Build history of the part. All positions in model axes, mm. A direction names the side the tool comes from. Give positions to 0.01 mm unless a question says otherwise; leave off trailing zeros. Write each loop counter-clockwise with the first axis right and the second up, starting at its lowest first coordinate (ties: lowest second). Pieces come first, ordered by that corner, then holes.
Autodesk Inventor part; units mm, degrees
ref_plane "YZ Plane" through (0, 0, 0) normal (1, 0, 0) x (0, 1, 0)
ref_plane "XZ Plane" through (0, 0, 0) normal (0, 1, 0) x (-1, 0, 0)
ref_plane "XY Plane" through (0, 0, 0) normal (0, 0, 1) x (1, 0, 0)
sketch "Sketch1" plane through (0, 0, 0) normal (0, 1, 0) x (-1, 0, 0)
  line L0 (0, 0) -> (100, 0)
  line L1 (100, 0) -> (100, -180)
  line L2 (100, -180) -> (0, -180)
  line L3 (0, -180) -> (0, 0)
  dimension "d0" = 100
  dimension "d1" = 180
sketch "Sketch2" plane through (0, 0, 0) normal (0, 1, 0) x (-1, 0, 0)
  circle A0 centre (49.0743, -61.8964) radius 10
  circle A1 centre (49.0743, -103.4918) radius 10
  circle A2 centre (49.0743, -145.129) radius 10
  line L0 (82.079, -27.0534) -> (82.079, -47.0534) construction
  line L1 (86.0942, -27.0534) -> (86.0942, -47.0534)
  line L2 (78.0638, -47.0534) -> (78.0638, -27.0534)
  arc A3 (86.0942, -27.0534) -> (78.0638, -27.0534) centre (82.079, -27.0534) ccw
  arc A4 (78.0638, -47.0534) -> (86.0942, -47.0534) centre (82.079, -47.0534) ccw
  line L3 (16.5655, -27.0534) -> (16.5655, -47.0534) construction
  line L4 (20.5808, -27.0534) -> (20.5808, -47.0534)
  line L5 (12.5503, -47.0534) -> (12.5503, -27.0534)
  arc A5 (20.5808, -27.0534) -> (12.5503, -27.0534) centre (16.5655, -27.0534) ccw
  arc A6 (12.5503, -47.0534) -> (20.5808, -47.0534) centre (16.5655, -47.0534) ccw
  line L6 (82.079, -138.3165) -> (82.079, -158.3165) construction
  line L7 (86.0942, -138.3165) -> (86.0942, -158.3165)
  line L8 (78.0638, -158.3165) -> (78.0638, -138.3165)
  arc A7 (86.0942, -138.3165) -> (78.0638, -138.3165) centre (82.079, -138.3165) ccw
  arc A8 (78.0638, -158.3165) -> (86.0942, -158.3165) centre (82.079, -158.3165) ccw
  line L9 (16.5655, -138.3165) -> (16.5655, -158.3165) construction
  line L10 (20.5808, -138.3165) -> (20.5808, -158.3165)
  line L11 (12.5503, -158.3165) -> (12.5503, -138.3165)
  arc A9 (20.5808, -138.3165) -> (12.5503, -138.3165) centre (16.5655, -138.3165) ccw
  arc A10 (12.5503, -158.3165) -> (20.5808, -158.3165) centre (16.5655, -158.3165) ccw
  point P0 (0, 0)
  point P1 (82.079, -37.0534)
  point P2 (16.5655, -37.0534)
  point P3 (82.079, -148.3165)
  point P4 (16.5655, -148.3165)
  dimension "d3" = 20
  dimension "d13" = 20
  dimension "d14" = 20
  dimension "d15" = 20
  dimension "d16" = 20
extrude "Extrusion1" add sketch "Sketch1" along normal blind 10
extrude "Extrusion2" cut sketch "Sketch2" along normal blind 10
sketch "Sketch6" plane through (0, 10, 0) normal (0, 1, 0) x (1, 0, 0)
  line L0 (-48.9569, 12.2049) -> (-48.9569, 32.2049) construction
  line L1 (-43.9569, 12.2049) -> (-43.9569, 32.2049)
  line L2 (-53.9569, 32.2049) -> (-53.9569, 12.2049)
  arc A0 (-53.9569, 12.2049) -> (-43.9569, 12.2049) centre (-48.9569, 12.2049) ccw
  arc A1 (-43.9569, 32.2049) -> (-53.9569, 32.2049) centre (-48.9569, 32.2049) ccw
  point P0 (0, 0)
  point P1 (-48.9569, 22.2049)
  dimension "d9" = 20
extrude "Extrusion3" cut sketch "Sketch6" against normal blind 10
properties part number "Sliding Plate"
1. Drill centre lines: line 1 along Z through (x, y) = (-51, 8.25); line 2 along Z through (x, y) = (-19, 5); line 3 along X through (y, z) = (1.25, -48.5). Where is each one in solid material? Low to high.
2. Mould opens along Z. For faces 1 (the face through (-43.957, 5, -22)), 2 (the face through (-100, 5, -89)), 3 (the face through (-51, 5, -180)) say: pulls with the +Z half, pulls with the -Z half, needs draft (parallel to the pull), parting line crosses it, or undercut.
3. 3-axis set-ups, long thin cutter, end or side, ignore diameter. For faces 4 (the face through (-49.067, 5.07, -7.206)), 5 (the face through (-49, 0, -89)): which of +Z, -Z, +X, -X, +Y, -Y reach the whole face in a straight line?
4. Saw through at A-A on z = -110. Give the cut face in (x, y), plus the area to 3 significant figures.
5. Saw through at B-B on y = 7. Count the separate pieces of the cut face and the enclosed holes in it, plus the area to 3 significant figures.
Outcome:
1. line 1: z = -180 to -154.94, -135.32 to -113.3, -93.68 to -71.71, -52.08 to -36.77, -7.64 to 0
1. line 2: z = -180 to -161.51, -135.12 to -50.25, -23.86 to 0
1. line 3: x = -100 to -85.82, -78.33 to -20.31, -12.82 to 0
2. face 1: undercut
2. face 2: needs draft
2. face 3: pulls with the -Z half
3. face 4: +Y, -Y
3. face 5: +Z, -Z, +X, -X, -Y
4. outline: (-100, 0) - (-56.67, 0) - (-56.67, 10) - (-100, 10) - close; (-41.48, 0) - (0, 0) - (0, 10) - (-41.48, 10) - close
4. area: 848 mm2
5. separate pieces: 1
5. enclosed holes: 8
5. area: 15,900 mm2
